Job drawing, mm, ordinate dimensions from the low corner. One solid piece. Coordinates: 2 decimals unless noted, no trailing zeros. Write each loop counter-clockwise with the first axis right and the second up, starting at its lowest first coordinate (ties: lowest second). Pieces come first, ordered by that corner, then holes.
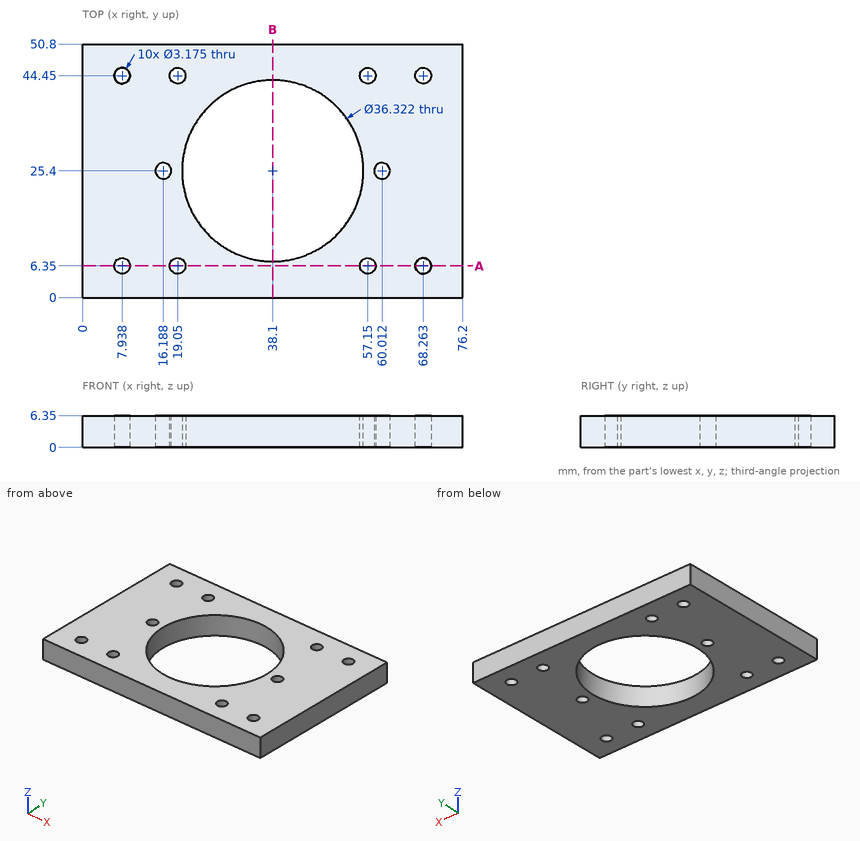
1. Saw through at B-B on x = 38.1. List the corners of the cut face in (y, z).
Computed values:
outline: (0, 0) - (7.24, 0) - (7.24, 6.35) - (0, 6.35) - close; (43.56, 0) - (50.8, 0) - (50.8, 6.35) - (43.56, 6.35) - close
2. Saw through at A-A on y = 6.35. State how many separate pieces and enclosed holes the cut face has, plus the area to 3 significant figures.
Computed values:
separate pieces: 5
enclosed holes: 0
area: 403 mm2
3. Probe line 1 along Y through (x, z) = (19.05, 2.5); line 2 along X through (y, z) = (44, 4.5) (1 decimal); line 3 along Y through (x, z) = (52.5, 3.5) (1 decimal). List the from-to ranges inside material, lowest first.
Computed values:
line 1: y = 0 to 4.76, 7.94 to 42.86, 46.04 to 50.8
line 2: x = 0 to 6.4, 9.5 to 17.5, 20.6 to 55.6, 58.7 to 66.7, 69.8 to 76.2
line 3: y = 0 to 14.3, 36.5 to 50.8
